Input: part model. Units: mm. Frame: model coordinates. A direction names the side the tool comes from. Give positions to 0.01 mm unless a question says otherwise; leave off trailing zeros. Loops run counter-clockwise (first coordinate to the right, second up) from the corner with the lowest first, then second, coordinate; pieces in that order, holes last. Notation, with made-up numbers: M 28,3 L 57,3 A29 cw 57,34 Z; hole C 40,-1 d2. An arc over 180 degrees is marked long. Use CSV: the item, a comma, the result in double quotes. Start each with the question number.
Q1. Section A-A, the plane z = 2.2. Output: boundary loops of the cut face in (x, y), plus the area to 3 significant figures.
Q2. Section C-C, the plane x = 669.5. Output: boundary loops of the cut face in (y, z), plus the area to 3 significant figures.
Q3. Reachability of faces 1 (the flat face through (546, -120, 3)), 2 (the flat face through (486, -326, 1.5)), 3 (the flat face through (717, -119, 1.5)) from +Z, -Z, +X, -X, +Y, -Y: full face, straight path, thin tool, end or side. Return the list, or none.
Q4. Pin query (flat end, axial travel): pin 1 (3.5 mm diameter, centred on x = 488.5, y = -325.5, fed in from +Z); pin 2 (3 mm diameter, centred on x = 504.31, y = -120.48, fed in from +Z); pin 3 (1.5 mm diameter, centred on x = 696, z = 2, fed in from -Y). Return the tip coordinate at first contact, or that it passes through.
Q5. Section B-B, the plane y = -274. Output: boundary loops of the cut face in (x, z), plus the area to 3 significant figures.
Q6. Material intervals for line 1 along X through (y, z) = (-190, 0.85); line 2 along Y through (x, z) = (667, 1.9), sorted ascending.
from build123d import *

# Parameters (mm, degrees)
CROQUIS3_R              = 1.75
SALIENTE_EXTRUIR1_DEPTH = 3
CORTAR_EXTRUIR1_START   = -1.5
CROQUIS4_W              = 7
CROQUIS4_H              = 10
CROQUIS4_R              = 1.75
CROQUIS4_W_2            = 10
CROQUIS4_H_2            = 7
CORTAR_EXTRUIR1_DEPTH   = 1.5


with BuildPart() as part:
    # Croquis3 → Saliente-Extruir1 (new body)
    with BuildSketch(Plane.XY):
        Polygon((483.811741117, -116.980180132), (483.811741117, -329.480180132), (490.811741117, -329.480180132), (490.811741117, -123.980180132), (720.611741117, -123.980180132), (720.611741117, -116.980180132), align=None)
        with Locations((487.311741117, -138.980180132)):
            Circle(CROQUIS3_R, mode=Mode.SUBTRACT)
        with Locations((487.311741117, -324.480180132)):
            Circle(CROQUIS3_R, mode=Mode.SUBTRACT)
        with Locations((504.311741117, -120.480180132)):
            Circle(CROQUIS3_R, mode=Mode.SUBTRACT)
        with Locations((715.611741117, -120.480180132)):
            Circle(CROQUIS3_R, mode=Mode.SUBTRACT)
    extrude(amount=SALIENTE_EXTRUIR1_DEPTH)

    # Croquis4 → Cortar-Extruir1 (cut)
    # profile 1 of 2: a face of its own
    with BuildSketch(Plane.XY.offset(3).offset(CORTAR_EXTRUIR1_START)):
        with Locations((487.311741117, -324.480180132)):
            Rectangle(CROQUIS4_W, CROQUIS4_H)
        with Locations((487.311741117, -324.480180132)):
            Circle(CROQUIS4_R, mode=Mode.SUBTRACT)
    # profile 2 of 2: a face of its own
    with BuildSketch(Plane.XY.offset(3).offset(CORTAR_EXTRUIR1_START)):
        with Locations((715.611741117, -120.480180132)):
            Rectangle(CROQUIS4_W_2, CROQUIS4_H_2)
        with Locations((715.611741117, -120.480180132)):
            Circle(CROQUIS4_R, mode=Mode.SUBTRACT)
    extrude(amount=CORTAR_EXTRUIR1_DEPTH, mode=Mode.SUBTRACT)


solid = part.part
A:
1,outline,"M 483.81,-319.48 L 490.81,-319.48 L 490.81,-123.98 L 710.61,-123.98 L 710.61,-116.98 L 483.81,-116.98 Z; hole C 487.31,-138.98 d3.5; hole C 504.31,-120.48 d3.5"
1,area,"2,940 mm^2"
2,outline,"M -123.98,0 L -116.98,0 L -116.98,3 L -123.98,3 Z"
2,area,"21.0 mm^2"
3,face 1,"+Z, +X, -X, +Y, -Y"
3,face 2,"+Z, +X, -X, -Y"
3,face 3,"+Z, +X, +Y, -Y"
4,pin 1,"z = 1.5"
4,pin 2,"through"
4,pin 3,"y = -123.98"
5,outline,"M 483.81,0 L 490.81,0 L 490.81,3 L 483.81,3 Z"
5,area,"21.0 mm^2"
6,line 1,"483.81 to 490.81"
6,line 2,"-123.98 to -116.98"
